Source: three-view drawing plus pictorial views. Frame: mm from the lowest corner of the part. A direction names the side the tool comes from. Give positions to 0.01 mm unless a question says otherwise; leave off trailing zeros. Loops run counter-clockwise (first coordinate to the right, second up) from the corner with the lowest first, then second, coordinate; pieces in that order, holes last.
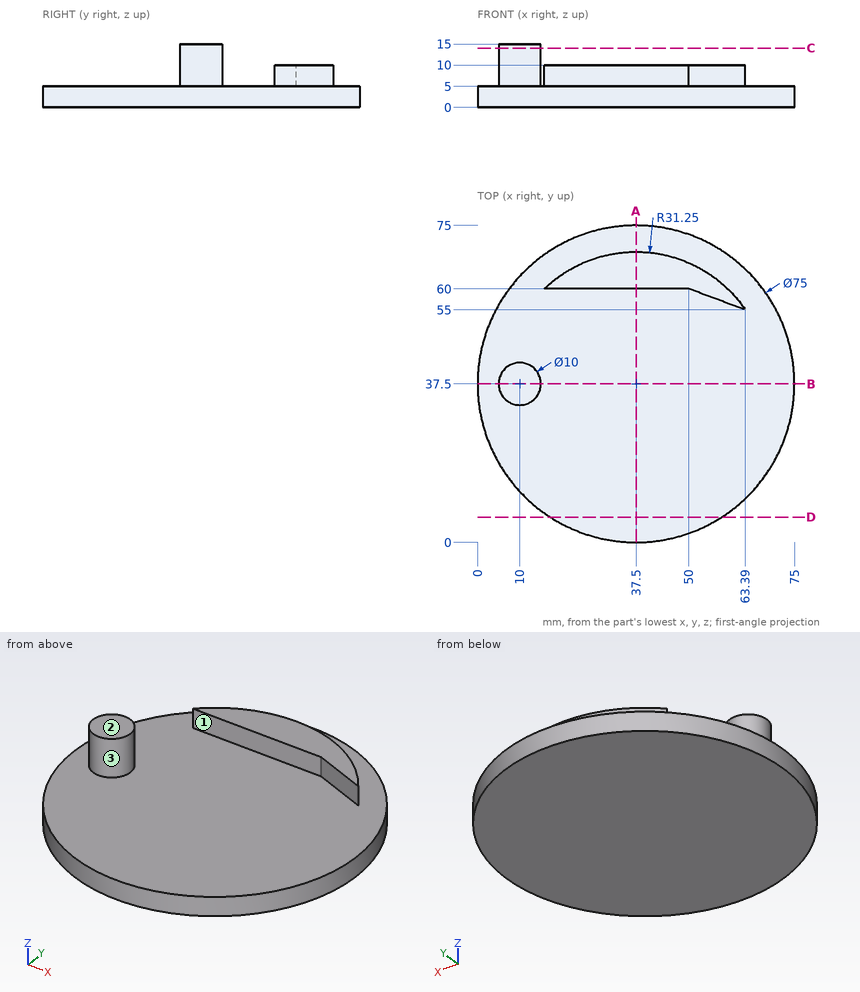
(1) Cut plane B-B (y = 37.5). Return the cut outline in (x, z), and give its area (3 significant figures).
Values follow:
outline: (0, 0) - (75, 0) - (75, 5) - (15, 5) - (15, 15) - (5, 15) - (5, 5) - (0, 5) - close
area: 475 mm2
(2) Cut plane C-C (z = 14). Return the cut outline in (x, y).
Values follow:
outline: circle Ø10 at (10, 37.5)
(3) Cut plane D-D (y = 6). Return the cut outline in (x, z).
Values follow:
outline: (17.15, 0) - (57.85, 0) - (57.85, 5) - (17.15, 5) - close
(4) Pin query (flat end, axial travel): pin 1 Ø15 at (x, y) = (41, 59) entering from +Z; pin 2 Ø22.5 at (x, y) = (43, 31) entering from +Z; pin 3 Ø5 at (x, z) = (38.5, 5.5) entering from -Y. Return the tip coordinate at first contact, or that it passes through.
Values follow:
pin 1: stops at z = 10
pin 2: stops at z = 5
pin 3: stops at y = 0
(5) Ray query, probe 1 along Z at (x, y) = (52, 57); probe 2 along X at (y, z) = (8, 2.5); probe 3 along Z at (x, y) = (33, 64). Return the intervals inside material, ascending.
Values follow:
probe 1: z = 0 to 5
probe 2: x = 14.35 to 60.65
probe 3: z = 0 to 10
(6) Reachability of the marked faces 1, 2 and 3 from +Z, -Z, +X, -X, +Y, -Y: full face, straight path, thin tool, end or side. Return the list, or none.
Values follow:
face 1: +Z, -X, -Y
face 2: +Z, +X, -X, +Y, -Y
face 3: +Z
(7) Cut plane A-A (x = 37.5). Return the cut outline in (y, z).
Values follow:
outline: (0, 0) - (75, 0) - (75, 5) - (68.75, 5) - (68.75, 10) - (60, 10) - (60, 5) - (0, 5) - close
